from build123d import *

# Parameters (mm, degrees)
CUT_EXTRUDE1_REACH = 43.911
SKETCH2_R          = 5.24
FILLET2_R          = 1
CHAMFER1_SIZE      = 0.5


# Read off the part's stored shape, not the designer's step: Draft1
with BuildPart() as part:
    # Sketch1 → Revolve1 (revolve)
    with BuildSketch(Plane.XY, mode=Mode.PRIVATE) as revolve1_sk:
        Polygon((0, 0), (9.765, 0), (9.765, -33), (12.5, -33), (12.5, -38), (0, -38), align=None)
    revolve(revolve1_sk.sketch.rotate(Axis((0, 5, 0), (0, -1, 0)), 180), axis=Axis((0, 5, 0), (0, -1, 0)))

    # Sketch2 → Cut-Extrude1 (cut, up to next)
    with BuildSketch(Plane(origin=(0, 0, 0), x_dir=(1, 0, 0), z_dir=(0, 1, 0)), mode=Mode.PRIVATE) as cut_extrude1_sk1:
        with Locations(Location((0, 0, 0), (0, 0, 180))):
            Circle(SKETCH2_R)
    cut_extrude1_tool1 = extrude(cut_extrude1_sk1.sketch, amount=-CUT_EXTRUDE1_REACH, mode=Mode.PRIVATE) & part.part
    add(cut_extrude1_tool1.solids().sort_by_distance((0, 0, 0))[0], mode=Mode.SUBTRACT)

    # Draft1 outline → Draft1 (revolve, cut)
    with BuildSketch(Plane.XY):
        Polygon((5.84743626, -38), (5.24, -3.2), (5.24, -38), align=None)
    revolve(axis=Axis((0, 0, 0), (0, 1, 0)), mode=Mode.SUBTRACT)

    # Fillet2
    fillet2_edges = [part.edges().sort_by_distance(p)[0] for p in [
        (9.765, -33, 0),
    ]]
    fillet(fillet2_edges, radius=FILLET2_R)

    # Chamfer1
    chamfer1_edges = [part.edges().sort_by_distance(p)[0] for p in [
        (12.5, -38, 0),
        (12.5, -33, 0),
    ]]
    chamfer(chamfer1_edges, length=CHAMFER1_SIZE)


solid = part.part
Can you work these out from the model? Positions are in its coordinate system, mm. A direction names the side the tool comes from. Round coordinates to 2 decimals unless told otherwise and drop trailing zeros. Order: outer loops, then holes, each group sorted by start corner. A loop starts at its lowest first (then second) coordinate and runs counter-clockwise, first axis right, second up. Notation, with made-up numbers: (36, -2) - (94, -2) arc R26 ccw to (94, 28) - close; hole circle Ø3 at (-37.5, 89.5). An arc over 180 degrees is marked (long way). Answer in a Markdown table with one row per item.
(1) Please list where these lines run through material, in increasing order: L1, parallel to Z at x = 0, y = -1.75 (3 decimals); L2, parallel to Y at x = -5.5, z = -10.25; L3, parallel to X at y = -34.5, z = -4. Write a range as from..to.
From the geometry:
| item | result |
|---|---|
| L1 | z = -9.765..-5.24, 5.24..9.765 |
| L2 | y = -38..-33 |
| L3 | x = -11.84..-4.18, 4.18..11.84 |
(2) Which directions (+Z, -Z, +X, -X, +Y, -Y) give clear straight access to the entire face, cutting with the end or side of a thin tool? Please do faces 1 (the face through (4, 0, 4)), 2 (the face through (-2, -33, 11)).
From the geometry:
| item | result |
|---|---|
| face 1 | +Z, -Z, +X, -X, +Y |
| face 2 | +Y |
(3) If we mould it in two halves opening along Z, with no side actions, what happens to faces 3 (the face through (-4.396, -20.356, 3.371)), 4 (the face through (6, -38, 2)), 5 (the face through (-9.314, -16.224, -2.933))? For each: released by +Z, released by -Z, zero draft, split by the parting line, or undercut.
From the geometry:
| item | result |
|---|---|
| face 3 | undercut |
| face 4 | zero draft |
| face 5 | split by the parting line |
(4) Suppose I cut it at A-A, the plane y = -22. Please give me the cut outline in (x, z) (3 decimals).
From the geometry:
| item | result |
|---|---|
| outline | circle Ø19.53 at (0, 0); hole circle Ø11.136 at (0, 0) |
(5) Suppose I cut it at B-B, the plane y = -28.5. Please give me the cut outline in (x, z) (3 decimals).
From the geometry:
| item | result |
|---|---|
| outline | circle Ø19.53 at (0, 0); hole circle Ø11.363 at (0, 0) |
(6) For P1, Ø1.5, axis at x = -0.5, y = -24, coming from the -Z side (3 decimals); P2, Ø3, axis at x = -9, y = -20, coming from the +Z side; P3, Ø3, axis at x = 3.5, y = -6.5, coming from the -Z side, each with a flat end and sliding along its axis, tell me the tip position at first contact or that it passes through.
From the geometry:
| item | result |
|---|---|
| P1 | stops at z = -9.765 |
| P2 | stops at z = 6.25 |
| P3 | stops at z = -9.56 |
